Geometry: final body of the model. Coordinates: model frame, mm. A direction names the side the tool comes from. Coordinates: 2 decimals unless noted, no trailing zeros. Loops run counter-clockwise (first coordinate to the right, second up) from the corner with the lowest first, then second, coordinate; pieces in that order, holes last. Notation, with made-up numbers: (63, -21.75) - (106, -21.75) arc R25 cw to (106, 3.25) - close; hole circle Ø1 at (56, 71). An arc over 180 degrees is marked (long way). Put each result on its own line as item: value. Start each with the question number.
1) Draft query along Y for faces 5 (the flat face through (0.07, 7.98, 2.84)), 6 (the flat face through (0, -7, 6.2)), 7 (the cylindrical face through (-1.22, -0.27, 4.54)). Return one class per face: +Y half, -Y half, draft (parallel to the pull), parting line (faces both ways), or undercut.
2) Contact query for flat-ended pins moving along their axis: pin 1 Ø0.9 at (x, z) = (-1.5, 8) entering from -Y; pin 2 Ø0.6 at (x, z) = (1, 0.5) entering from -Y; pin 3 Ø1 at (x, z) = (-0.5, 1) entering from +Y. Output: stop coordinate, or through.
3) Reachability of faces 1 (the flat face through (0, -6.5, 1)), 2 (the flat face through (0, 7, 6.2)), 3 (the flat face through (0, -4, 8)), 4 (the flat face through (0, 6.5, 1)) from +Z, -Z, +X, -X, +Y, -Y: full face, straight path, thin tool, end or side. Return the list, or none.
4) Material intervals for line 1 along X through (y, z) = (0, 3.75); line 2 along Z through (x, y) = (-0.25, 3.75); line 3 along Z through (x, y) = (-1, -6.75), sorted ascending. Write a range as from..to.
5) Section C-C on y = 6.25. Output: boundary loops of the cut face in (x, z), and give its area (3 significant figures).
```python
from build123d import *

# Parameters (mm, degrees)
PAD005_DEPTH    = 5
POCKET002_DEPTH = 0.001
SKETCH010_R     = 1.25
POCKET003_DEPTH = 9.2


with BuildPart() as part:
    # Sketch008 → Pad005 (new body, symmetric)
    with BuildSketch(Plane.YZ):
        Polygon((-6.5, 0), (-6.5, 2), (-9.5, 3.7), (-9.5, 6.2), (-4, 6.2), (-4, 9.2), (0, 9.2), (0, 0), align=None)
    pad005 = extrude(amount=PAD005_DEPTH, both=True)

    # Mirrored: Pad005 across Sketch008 V_Axis
    add(pad005.mirror(Plane(origin=(0, 0, 0), x_dir=(1, 0, 0), z_dir=(0, 1, 0))))

    # Sketch009 (on Face2 of Mirrored) → Pocket002 (cut)
    with BuildSketch(Plane.YX):
        Polygon((-2.136196, 3.7), (-4.272392, 0), (-2.136196, -3.7), (2.136196, -3.7), (4.272392, 0), (2.136196, 3.7), align=None)
    extrude(amount=-POCKET002_DEPTH, mode=Mode.SUBTRACT)

    # Sketch010 (on Face20 of Pocket002) → Pocket003 (cut, through all)
    with BuildSketch(Plane.YX.offset(-0.001)):
        Circle(SKETCH010_R)
    extrude(amount=-POCKET003_DEPTH, mode=Mode.SUBTRACT)


solid = part.part
```
Answer block:
1. face 5: +Y half
1. face 6: draft
1. face 7: undercut
2. pin 1: stops at y = -4
2. pin 2: stops at y = -6.5
2. pin 3: stops at y = 6.5
3. face 1: -Z, +X, -X, -Y
3. face 2: +Z, +X, -X, +Y
3. face 3: +Z, +X, -X, -Y
3. face 4: -Z, +X, -X, +Y
4. line 1: x = -5..-1.25, 1.25..5
4. line 2: z = 0..9.2
4. line 3: z = 2.14..6.2
5. outline: (-5, 0) - (5, 0) - (5, 6.2) - (-5, 6.2) - close
5. area: 62.0 mm²
